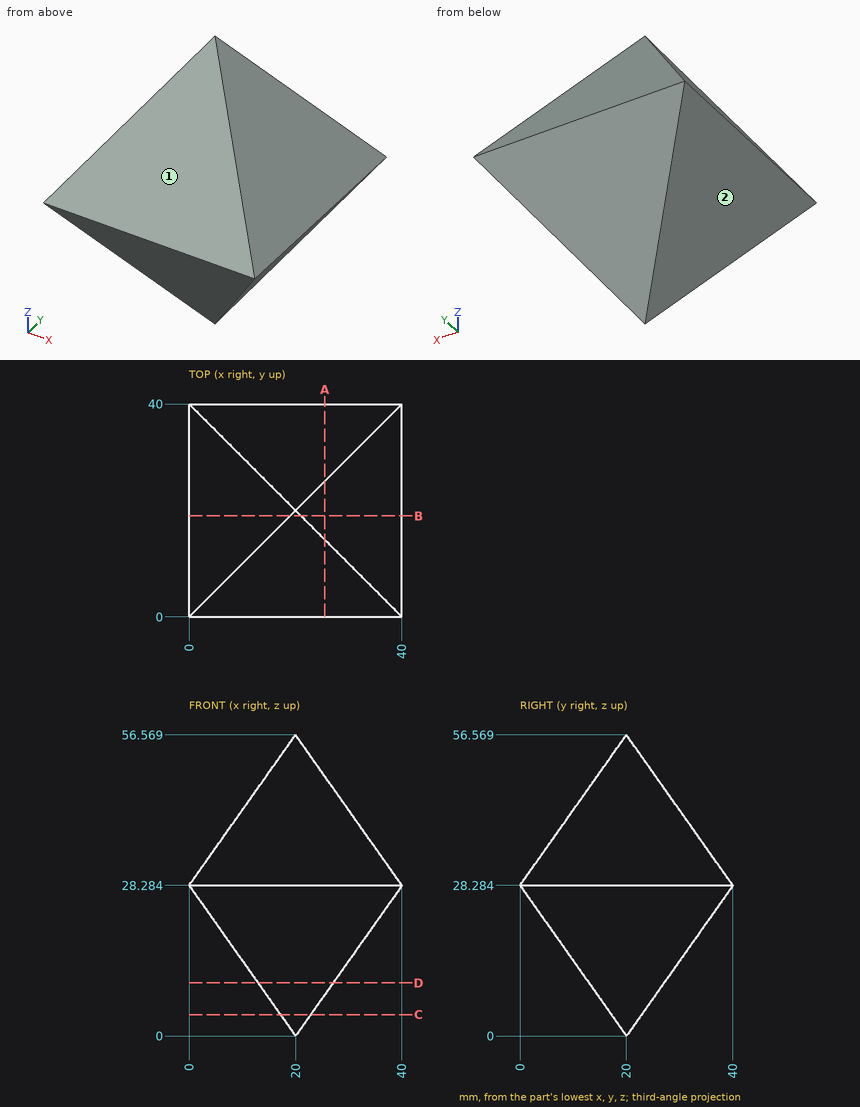
Geometry check sheet. Reference: drawing and pictorial views, mm from the part's lowest x, y, z. Give positions to 0.01 mm unless a question says otherwise; leave off trailing zeros. Loops run counter-clockwise (first coordinate to the right, second up) from the corner with the lowest first, then second, coordinate; pieces in that order, holes last. Notation, with made-up numbers: (57.25, 25.25) -> (84.25, 25.25) arc R21 cw to (84.25, 45.25) -> close; hole circle Ø5 at (-1.5, 35). An arc over 180 degrees is marked (long way). Answer in a Markdown table with one row per item. Add a question column.
1) Material ranges on probe 1 along X at (y, z) = (20.5, 7.5) (1 decimal); probe 2 along Z at (x, y) = (36.5, 20) (1 decimal); probe 3 along Z at (x, y) = (18.5, 34.5) (1 decimal), recorded low to high. Write a range as from..to.
2) Cross-section at C-C on z = 4. Record the boundary of the cut face in (x, y), and give its area (3 significant figures).
3) Cross-section at D-D on z = 10. Record the boundary of the cut face in (x, y).
4) Gauge pin test, flat ends, axial feed: P1, Ø3, axis at x = 7.5, z = 21.5, coming from the -Y side; P2, Ø2, axis at x = 33, z = 35.5, coming from the +Y side (1 decimal); P3, Ø3, axis at x = 14, y = 18.5, coming from the -Z side (1 decimal). Record the tip position at first contact, or that the pin passes through.
5) Cross-section at B-B on y = 19. Record the boundary of the cut face in (x, z) (1 decimal), and give its area (3 significant figures).
6) Draft check along Z on the marked faces 1 and 2. Enter one of: pulls with the +Z half, pulls with the -Z half, needs draft (parallel to the pull), parting line crosses it, or undercut.
7) Cross-section at A-A on x = 25.5. Record the boundary of the cut face in (y, z) (1 decimal).
Outcome:
| question | item | result |
|---|---|---|
| 1 | probe 1 | x = 14.7..25.3 |
| 1 | probe 2 | z = 23.3..33.2 |
| 1 | probe 3 | z = 20.5..36.1 |
| 2 | outline | (17.17, 17.17) -> (22.83, 17.17) -> (22.83, 22.83) -> (17.17, 22.83) -> close |
| 2 | area | 32.0 mm^2 |
| 3 | outline | (12.93, 12.93) -> (27.07, 12.93) -> (27.07, 27.07) -> (12.93, 27.07) -> close |
| 4 | P1 | stops at y = 3.74 |
| 4 | P2 | stops at y = 35.6 |
| 4 | P3 | stops at z = 6.4 |
| 5 | outline | (0, 28.3) -> (19, 1.4) -> (21, 1.4) -> (40, 28.3) -> (21, 55.2) -> (19, 55.2) -> close |
| 5 | area | 1,130 mm^2 |
| 6 | face 1 | pulls with the +Z half |
| 6 | face 2 | pulls with the -Z half |
| 7 | outline | (0, 28.3) -> (14.5, 7.8) -> (25.5, 7.8) -> (40, 28.3) -> (25.5, 48.8) -> (14.5, 48.8) -> close |
